from build123d import *

# Parameters (mm, degrees)
SKETCH_1_W          = 120
SKETCH_1_H          = 190
SKETCH_1_R          = 4.25
SKETCH_1_W_2        = 90
SKETCH_1_H_2        = 80
EXTRUDE_1_DEPTH     = 8
SKETCH_2_W          = 102
SKETCH_2_H          = 92
SKETCH_2_W_2        = 90
SKETCH_2_H_2        = 80
EXTRUDE_2_DEPTH     = 70
SKETCH_3_R          = 4.25
CUT_EXTRUDE_1_DEPTH = 145.637477854
FILLET_1_R          = 3


with BuildPart() as part:
    # 草图1 → 凸台-拉伸1 (new body)
    with BuildSketch(Plane(origin=(0, 0, 0), x_dir=(1, 0, 0), z_dir=(0, 1, 0))):
        Rectangle(SKETCH_1_W, SKETCH_1_H)
        with Locations(Location((20, 85, 0), (0, 0, 270))):
            Circle(SKETCH_1_R, mode=Mode.SUBTRACT)
        with Locations(Location((20, 25, 0), (0, 0, 270))):
            Circle(SKETCH_1_R, mode=Mode.SUBTRACT)
        with Locations(Location((-20, 85, 0), (0, 0, 90))):
            Circle(SKETCH_1_R, mode=Mode.SUBTRACT)
        with Locations(Location((-20, 25, 0), (0, 0, 90))):
            Circle(SKETCH_1_R, mode=Mode.SUBTRACT)
        with Locations((0, -35)):
            Rectangle(SKETCH_1_W_2, SKETCH_1_H_2, mode=Mode.SUBTRACT)
    extrude(amount=EXTRUDE_1_DEPTH)

    # 草图2 → 凸台-拉伸2 (add)
    with BuildSketch(Plane(origin=(0, 8, 0), x_dir=(1, 0, 0), z_dir=(0, 1, 0))):
        with Locations((0, -35)):
            Rectangle(SKETCH_2_W, SKETCH_2_H)
        with Locations((0, -35)):
            Rectangle(SKETCH_2_W_2, SKETCH_2_H_2, mode=Mode.SUBTRACT)
    extrude(amount=EXTRUDE_2_DEPTH)

    # 草图3 → 切除-拉伸1 (cut, through all)
    with BuildSketch(Plane(origin=(0, 0, -11), x_dir=(-1, 0, 0), z_dir=(0, 0, -1))):
        with Locations((20, 68)):
            Circle(SKETCH_3_R)
        with Locations((20, 38)):
            Circle(SKETCH_3_R)
        with Locations(Location((-20, 38, 0), (0, 0, 180))):
            Circle(SKETCH_3_R)
        with Locations(Location((-20, 68, 0), (0, 0, 180))):
            Circle(SKETCH_3_R)
    extrude(amount=-CUT_EXTRUDE_1_DEPTH, mode=Mode.SUBTRACT)

    # 圆角1
    fillet_1_edges = [part.edges().sort_by_distance(p)[0] for p in [
        (-45, 39, -5),
        (-45, 39, 75),
        (45, 39, 75),
        (45, 39, -5),
    ]]
    fillet(fillet_1_edges, radius=FILLET_1_R)


solid = part.part
For this review, take the finished solid that the model builds, in its own axes (mm). A direction names the side the tool comes from. Coordinates: 2 decimals unless noted, no trailing zeros. Order: outer loops, then holes, each group sorted by start corner. A loop starts at its lowest first (then second) coordinate and runs counter-clockwise, first axis right, second up. Notation, with made-up numbers: (17, 36) -> (55, 36) arc R26 ccw to (55, 60) -> close; hole circle Ø8 at (19.5, 85). An arc over 180 degrees is marked (long way). Return JSON: item names as keys, results as strings.
1. We need section A-A on z = -85. Write out the cut boundary in (x, y).
Answer block:
{"outline": "(-60, 0) -> (-24.25, 0) -> (-24.25, 8) -> (-60, 8) -> close; (-15.75, 0) -> (15.75, 0) -> (15.75, 8) -> (-15.75, 8) -> close; (24.25, 0) -> (60, 0) -> (60, 8) -> (24.25, 8) -> close"}
2. Machinability: for faces 1 (the flat face through (-1, 43, 81)), 2 (the flat face through (-1, 43, -11)), 3 (the flat face through (51, 43, 36)), 4 (the cylindrical face through (19.447, 33.786, -8.042)), 5 (the flat face through (-1, 38, 75)), which of the approach directions +Z, -Z, +X, -X, +Y, -Y give a long, thin tool a straight path to every point of the face, cutting with its end or side? Answer none if there is none.
Answer block:
{"face 1": "+Z, +X, -X, +Y", "face 2": "-Z, +X, -X, +Y", "face 3": "+Z, -Z, +X, +Y", "face 4": "+Z, -Z", "face 5": "+Y, -Y"}
3. The part is to be moulded in two halves that separate along Y. For faces 6 (the cylindrical face through (21.96, 71.77, 77.96)), 7 (the flat face through (-1, 0, -22)), 8 (the cylindrical face through (17.41, 3.94, -28.37)), say which applies: +Y half, -Y half, draft (parallel to the pull), parting line (faces both ways), or undercut.
Answer block:
{"face 6": "undercut", "face 7": "-Y half", "face 8": "draft"}
4. We need section B-B on y = 11.5. Write out the cut boundary in (x, z), and give its area (3 significant figures).
Answer block:
{"outline": "(-51, -11) -> (51, -11) -> (51, 81) -> (-51, 81) -> close; hole (-45, -2) arc R3 ccw to (-42, -5) -> (42, -5) arc R3 ccw to (45, -2) -> (45, 72) arc R3 ccw to (42, 75) -> (-42, 75) arc R3 ccw to (-45, 72) -> close", "area": "2,190 mm²"}
5. For line 1 (Y direction, x = -20, z = -6.4); line 2 (X direction, y = 3, z = -85); line 3 (Z direction, x = -20, y = 5.75), list the stretches that pass through material, from the lowest coordinate up. Write a range as from..to.
Answer block:
{"line 1": "0..33.75, 42.25..63.75, 72.25..78", "line 2": "-60..-24.25, -15.75..15.75, 24.25..60", "line 3": "-95..-89.25, -80.75..-29.25, -20.75..-5, 75..95"}
6. We need section C-C on x = -38.5. Write out the cut boundary in (y, z).
Answer block:
{"outline": "(0, -95) -> (8, -95) -> (8, -11) -> (78, -11) -> (78, -5) -> (0, -5) -> close; (0, 75) -> (78, 75) -> (78, 81) -> (8, 81) -> (8, 95) -> (0, 95) -> close"}
7. We need section D-D on z = 23. Write out the cut boundary in (x, y).
Answer block:
{"outline": "(-60, 0) -> (-45, 0) -> (-45, 78) -> (-51, 78) -> (-51, 8) -> (-60, 8) -> close; (45, 0) -> (60, 0) -> (60, 8) -> (51, 8) -> (51, 78) -> (45, 78) -> close"}
8. For pin 1 Ø11 at (x, y) = (20, 38) entering from +Z; pin 2 Ø8 at (y, z) = (29.5, 62.5) entering from -X; pin 3 Ø10 at (x, z) = (-20, -25) entering from +Y; pin 4 Ø2 at (x, z) = (37.5, -23.5) entering from -Y, all flat-tipped, find the tip position at first contact; note any pin that passes through.
Answer block:
{"pin 1": "z = 81", "pin 2": "x = -51", "pin 3": "y = 8", "pin 4": "y = 0"}
